Part print with two shaded views. Sizes in mm from the minimum x, y, z corner. A direction names the side the tool comes from. Round coordinates to 2 decimals unless told otherwise and drop trailing zeros. Write each loop counter-clockwise with the first axis right and the second up, starting at its lowest first coordinate (ties: lowest second). Pieces come first, ordered by that corner, then holes. Notation, with made-up numbers: (80, 52) -> (90, 52) arc R24 ccw to (90, 78) -> close; hole circle Ø6 at (-35.75, -25.75). An arc over 180 degrees is marked (long way). Put each result on its own line as item: value. Start each with the question number.
1. Saw through at A-A on y = 101.6. List the corners of the cut face in (x, z), and give its area (3 significant figures).
2. Flat gauge pins, fed straight in: P1, Ø1, axis at y = 65.5, z = 24.5, coming from the -X side; P2, Ø10, axis at x = 55, z = 11.5, coming from the +Y side; P3, Ø1.5, axis at x = 55, y = 92.5, coming from the -Z side. Where does each tip first touch, or does it go through?
3. 3-axis set-ups, long thin cutter, end or side, ignore diameter. For the marked faces 1 and 2: which of +Z, -Z, +X, -X, +Y, -Y reach the whole face in a straight line?
4. Saw through at D-D on x = 67. List the corners of the cut face in (y, z).
5. Drill centre line: line 1 (Z direction, x = 10.5, y = 87.5). Where is it in solid material? Low to high. Write a range as from..to.
6. Saw through at B-B on x = 44.45. List the corners of the cut face in (y, z), and give its area (3 significant figures).
7. Saw through at C-C on z = 7.5. List the corners of the cut face in (x, y).
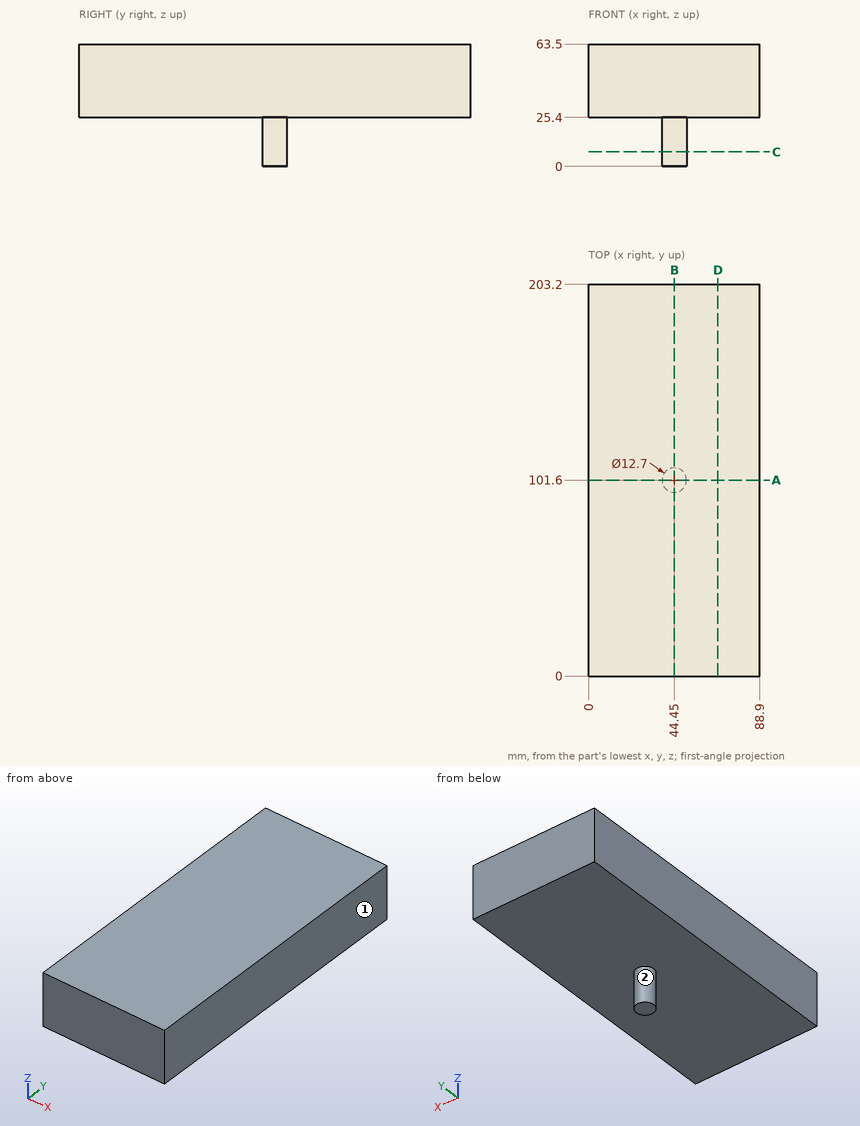
Return value:
1. outline: (0, 25.4) -> (38.1, 25.4) -> (38.1, 0) -> (50.8, 0) -> (50.8, 25.4) -> (88.9, 25.4) -> (88.9, 63.5) -> (0, 63.5) -> close
1. area: 3,710 mm^2
2. P1: passes through
2. P2: stops at y = 104.69
2. P3: stops at z = 25.4
3. face 1: +Z, -Z, +X, +Y, -Y
3. face 2: -Z
4. outline: (0, 25.4) -> (203.2, 25.4) -> (203.2, 63.5) -> (0, 63.5) -> close
5. line 1: z = 25.4..63.5
6. outline: (0, 25.4) -> (95.25, 25.4) -> (95.25, 0) -> (107.95, 0) -> (107.95, 25.4) -> (203.2, 25.4) -> (203.2, 63.5) -> (0, 63.5) -> close
6. area: 8,060 mm^2
7. outline: circle Ø12.7 at (44.45, 101.6)
